Part model, mm, in its own coordinate system. Coordinates: 2 decimals unless noted, no trailing zeros. Order: outer loops, then holes, each group sorted by start corner. A loop starts at its lowest first (then second) coordinate and runs counter-clockwise, first axis right, second up.
1) Cut at C-C (x = -89.5). List the corners of the cut face in (y, z), and give its area (3 significant figures).
2) Wall check: L1, parallel to X at y = 0.4, z = 13.5; L2, parallel to X at y = 2.1, z = -13.5; L3, parallel to X at y = 2.65, z = 7. Give the ranges that are in metal, low to high.
3) Pin check, flat tips, straight feed: pin 1 Ø1.5 at (x, y) = (-113, 2) entering from +Z; pin 2 Ø12 at (x, z) = (-74.5, -11.5) entering from -Y; pin 3 Ø3 at (x, z) = (-105.57, -13.5) entering from +Y; pin 4 Ø1 at (y, z) = (1.5, -20) entering from -X. Stop position of each tip, or through.
4) Cut at A-A (z = -4.5). List the corners of the cut face in (x, y), and give its area (3 significant figures).
5) Cut at B-B (y = 1.8). Give the number of separate pieces and of enclosed holes in the cut face, and give its area (3 significant figures).
```python
from build123d import *

# Parameters (mm, degrees)
EXTRUDE_1_DEPTH              = 3
CUT_EXTRUDE_1_REACH          = 217.134
HOLE_WIZARD_M2_2_D           = 2.4
HOLE_WIZARD_M2_2_CBORE_D     = 4.4
HOLE_WIZARD_M2_2_CBORE_DEPTH = 2
CUT_EXTRUDE_2_REACH          = 217.134
HOLE_WIZARD_M2_3_D           = 2.4
HOLE_WIZARD_M2_3_CBORE_D     = 4.4
HOLE_WIZARD_M2_3_CBORE_DEPTH = 2
MIRROR_7_COPY_1_REACH        = 217.134
MIRROR_7_COPY_2_D            = 2.4
MIRROR_7_COPY_2_CBORE_D      = 4.4
MIRROR_7_COPY_2_CBORE_DEPTH  = 2
CUT_EXTRUDE_3_REACH          = 217.134
SKETCH_18_W                  = 20
SKETCH_18_H                  = 10
HOLE_WIZARD_M2_4_D           = 2.4
HOLE_WIZARD_M2_4_CBORE_D     = 4.4
HOLE_WIZARD_M2_4_CBORE_DEPTH = 2
HOLE_WIZARD_M2_5_D           = 2.4
HOLE_WIZARD_M2_5_CBORE_D     = 4.4
HOLE_WIZARD_M2_5_CBORE_DEPTH = 2
HOLE_WIZARD_M2_6_D           = 2.4
HOLE_WIZARD_M2_6_CBORE_D     = 4.4
HOLE_WIZARD_M2_6_CBORE_DEPTH = 2
SKETCH_24_W                  = 20
SKETCH_24_H                  = 56
CUT_EXTRUDE_4_DEPTH          = 10
HOLE_WIZARD_M2_7_D           = 2.4
HOLE_WIZARD_M2_7_CBORE_D     = 4.4
HOLE_WIZARD_M2_7_CBORE_DEPTH = 2
SKETCH_26_OUTSIDE_W          = 390.69
SKETCH_26_OUTSIDE_H          = 393.83
SKETCH_26_OUTSIDE_W_2        = 151.320508076
SKETCH_26_OUTSIDE_H_2        = 56
CUT_EXTRUDE_6_DEPTH          = 10


with BuildPart() as part:
    # 草图1 → 凸台-拉伸1 (new body)
    with BuildSketch(Plane(origin=(0, 0, 0), x_dir=(1, 0, 0), z_dir=(0, 1, 0))):
        Polygon((-45.715728753, 114), (45.715728753, 114), (84.606601718, 152.890872965), (91.67766953, 152.890872965), (112.890872965, 131.67766953), (112.890872965, 124.606601718), (74, 85.715728753), (74, 30), (91.320508076, 20), (146.320508076, 20), (151.320508076, 15), (151.320508076, -15), (146.320508076, -20), (91.320508076, -20), (74, -30), (74, -85.715728753), (112.890872965, -124.606601718), (112.890872965, -131.67766953), (91.67766953, -152.890872965), (84.606601718, -152.890872965), (45.715728753, -114), (-45.715728753, -114), (-84.606601718, -152.890872965), (-91.67766953, -152.890872965), (-112.890872965, -131.67766953), (-112.890872965, -124.606601718), (-74, -85.715728753), (-74, -30), (-91.320508076, -20), (-146.320508076, -20), (-151.320508076, -15), (-151.320508076, 15), (-146.320508076, 20), (-91.320508076, 20), (-74, 30), (-74, 85.715728753), (-112.890872965, 124.606601718), (-112.890872965, 131.67766953), (-91.67766953, 152.890872965), (-84.606601718, 152.890872965), align=None)
    extrude(amount=EXTRUDE_1_DEPTH)

    # 草图2 → 切除-拉伸1 (cut, up to next)
    with BuildSketch(Plane(origin=(0, 3, 0), x_dir=(1, 0, 0), z_dir=(0, 1, 0)), mode=Mode.PRIVATE) as cut_extrude_1_sk1:
        with BuildLine():
            Line((103.820508076, -10), (103.820508076, 10))
            Line((103.820508076, 10), (129.687258495, 10))
            ThreePointArc((129.687258495, 10), (148.320508076, 0), (129.687258495, -10))
            Line((129.687258495, -10), (103.820508076, -10))
        make_face()
    cut_extrude_1_tool1 = extrude(cut_extrude_1_sk1.sketch, amount=-CUT_EXTRUDE_1_REACH, mode=Mode.PRIVATE) & part.part
    cut_extrude_1 = cut_extrude_1_tool1.solids().sort_by_distance((125.74589, 3, 0))[0]
    add(cut_extrude_1, mode=Mode.SUBTRACT)

    # M2 凹头盖螺钉的柱形沉头孔2 (through all)
    with Locations(Plane(origin=(100.320508076, 3, -8), x_dir=(0, 0, 1), z_dir=(0, 1, 0))):
        with Locations((0, 0), (-5.5, 5.25), (-5.5, 13.25), (-5.5, 21.25), (-5.5, 29.25), (16, 0), (21.5, 5.25), (21.5, 13.25), (21.5, 21.25), (21.5, 29.25)):
            hole_wizard_m2_2 = CounterBoreHole(HOLE_WIZARD_M2_2_D / 2, HOLE_WIZARD_M2_2_CBORE_D / 2, HOLE_WIZARD_M2_2_CBORE_DEPTH)

    # 草图10 → 切除-拉伸2 (cut, up to next)
    with BuildSketch(Plane(origin=(0, 3, 0), x_dir=(1, 0, 0), z_dir=(0, 1, 0)), mode=Mode.PRIVATE) as cut_extrude_2_sk1:
        with BuildLine():
            Line((75.767766953, 101.625631329), (61.625631329, 115.767766953))
            Line((61.625631329, 115.767766953), (79.916185958, 134.058321582))
            ThreePointArc((79.916185958, 134.058321582), (100.162950904, 140.162950904), (94.058321582, 119.916185958))
            Line((94.058321582, 119.916185958), (75.767766953, 101.625631329))
        make_face()
    cut_extrude_2_tool1 = extrude(cut_extrude_2_sk1.sketch, amount=-CUT_EXTRUDE_2_REACH, mode=Mode.PRIVATE) & part.part
    cut_extrude_2 = cut_extrude_2_tool1.solids().sort_by_distance((84.200285, 3, -124.200285))[0]
    add(cut_extrude_2, mode=Mode.SUBTRACT)

    # M2 凹头盖螺钉的柱形沉头孔3 (through all)
    with Locations(Plane(origin=(60.388194462, 3, -119.480077554), x_dir=(0, 0, 1), z_dir=(0, 1, 0))):
        with Locations((0, 0), (-5.65685425, 5.65685425), (-11.313708499, 11.313708499), (-16.970562749, 16.970562749), (7.601397898, 0.176776695), (18.915106397, 11.490485194), (19.091883092, 19.091883092), (13.435028842, 24.748737342), (7.778174593, 30.405591591), (2.121320343, 36.062445841)):
            hole_wizard_m2_3 = CounterBoreHole(HOLE_WIZARD_M2_3_D / 2, HOLE_WIZARD_M2_3_CBORE_D / 2, HOLE_WIZARD_M2_3_CBORE_DEPTH)

    # 镜向5: 切除-拉伸1, M2 凹头盖螺钉的柱形沉头孔2 across plane
    add(cut_extrude_1.mirror(Plane(origin=(0, 0, 0), x_dir=(0, 0, 1), z_dir=(1, 0, 0))), mode=Mode.SUBTRACT)
    add(hole_wizard_m2_2.mirror(Plane(origin=(0, 0, 0), x_dir=(0, 0, 1), z_dir=(1, 0, 0))), mode=Mode.SUBTRACT)

    # 镜向6: 切除-拉伸2, M2 凹头盖螺钉的柱形沉头孔3 across plane
    add(cut_extrude_2.mirror(Plane(origin=(0, 0, 0), x_dir=(0, 0, 1), z_dir=(1, 0, 0))), mode=Mode.SUBTRACT)
    add(hole_wizard_m2_3.mirror(Plane(origin=(0, 0, 0), x_dir=(0, 0, 1), z_dir=(1, 0, 0))), mode=Mode.SUBTRACT)

    # 镜向7: 切除-拉伸2, M2 凹头盖螺钉的柱形沉头孔3 across plane
    add(cut_extrude_2.mirror(Plane.XY), mode=Mode.SUBTRACT)
    add(hole_wizard_m2_3.mirror(Plane.XY), mode=Mode.SUBTRACT)

    # 镜向7 copy 1 sketch → 镜向7 copy 1 (cut, up to next)
    with BuildSketch(Plane(origin=(0, 3, 0), x_dir=(-1, 0, 0), z_dir=(0, 1, 0)), mode=Mode.PRIVATE) as mirror_7_copy_1_sk1:
        with BuildLine():
            Line((75.767766953, 101.625631329), (61.625631329, 115.767766953))
            Line((61.625631329, 115.767766953), (79.916185958, 134.058321582))
            ThreePointArc((79.916185958, 134.058321582), (100.162950904, 140.162950904), (94.058321582, 119.916185958))
            Line((94.058321582, 119.916185958), (75.767766953, 101.625631329))
        make_face()
    mirror_7_copy_1_tool1 = extrude(mirror_7_copy_1_sk1.sketch, amount=-MIRROR_7_COPY_1_REACH, mode=Mode.PRIVATE) & part.part
    add(mirror_7_copy_1_tool1.solids().sort_by_distance((-84.200285, 3, 124.200285))[0], mode=Mode.SUBTRACT)

    # 镜向7 copy 2 (through all)
    with Locations(Plane(origin=(-60.388194462, 3, 119.480077554), x_dir=(0, 0, -1), z_dir=(0, 1, 0))):
        with Locations((0, 0), (-5.65685425, 5.65685425), (-11.313708499, 11.313708499), (-16.970562749, 16.970562749), (7.601397898, 0.176776695), (18.915106397, 11.490485194), (19.091883092, 19.091883092), (13.435028842, 24.748737342), (7.778174593, 30.405591591), (2.121320343, 36.062445841)):
            CounterBoreHole(MIRROR_7_COPY_2_D / 2, MIRROR_7_COPY_2_CBORE_D / 2, MIRROR_7_COPY_2_CBORE_DEPTH)

    # 草图18 → 切除-拉伸3 (cut, up to next)
    with BuildSketch(Plane(origin=(0, 3, 0), x_dir=(1, 0, 0), z_dir=(0, 1, 0)), mode=Mode.PRIVATE) as cut_extrude_3_sk1:
        Polygon((-60, -28), (-15, -28), (-15, -63), (-60, -83), align=None)
    cut_extrude_3_tool1 = extrude(cut_extrude_3_sk1.sketch, amount=-CUT_EXTRUDE_3_REACH, mode=Mode.PRIVATE) & part.part
    # 草图18 → 切除-拉伸3 (cut, up to next)
    with BuildSketch(Plane(origin=(0, 3, 0), x_dir=(1, 0, 0), z_dir=(0, 1, 0)), mode=Mode.PRIVATE) as cut_extrude_3_sk2:
        with Locations((20, -99)):
            Rectangle(SKETCH_18_W, SKETCH_18_H)
    cut_extrude_3_tool2 = extrude(cut_extrude_3_sk2.sketch, amount=-CUT_EXTRUDE_3_REACH, mode=Mode.PRIVATE) & part.part
    # 草图18 → 切除-拉伸3 (cut, up to next)
    with BuildSketch(Plane(origin=(0, 3, 0), x_dir=(1, 0, 0), z_dir=(0, 1, 0)), mode=Mode.PRIVATE) as cut_extrude_3_sk3:
        with Locations((-20, -99)):
            Rectangle(SKETCH_18_W, SKETCH_18_H)
    cut_extrude_3_tool3 = extrude(cut_extrude_3_sk3.sketch, amount=-CUT_EXTRUDE_3_REACH, mode=Mode.PRIVATE) & part.part
    # 草图18 → 切除-拉伸3 (cut, up to next)
    with BuildSketch(Plane(origin=(0, 3, 0), x_dir=(1, 0, 0), z_dir=(0, 1, 0)), mode=Mode.PRIVATE) as cut_extrude_3_sk4:
        Polygon((15, -63), (60, -83), (60, -28), (15, -28), align=None)
    cut_extrude_3_tool4 = extrude(cut_extrude_3_sk4.sketch, amount=-CUT_EXTRUDE_3_REACH, mode=Mode.PRIVATE) & part.part
    # 草图18 → 切除-拉伸3 (cut, up to next)
    with BuildSketch(Plane(origin=(0, 3, 0), x_dir=(1, 0, 0), z_dir=(0, 1, 0)), mode=Mode.PRIVATE) as cut_extrude_3_sk5:
        with Locations((-20, 99)):
            Rectangle(SKETCH_18_W, SKETCH_18_H)
    cut_extrude_3_tool5 = extrude(cut_extrude_3_sk5.sketch, amount=-CUT_EXTRUDE_3_REACH, mode=Mode.PRIVATE) & part.part
    # 草图18 → 切除-拉伸3 (cut, up to next)
    with BuildSketch(Plane(origin=(0, 3, 0), x_dir=(1, 0, 0), z_dir=(0, 1, 0)), mode=Mode.PRIVATE) as cut_extrude_3_sk6:
        with Locations((20, 99)):
            Rectangle(SKETCH_18_W, SKETCH_18_H)
    cut_extrude_3_tool6 = extrude(cut_extrude_3_sk6.sketch, amount=-CUT_EXTRUDE_3_REACH, mode=Mode.PRIVATE) & part.part
    # 草图18 → 切除-拉伸3 (cut, up to next)
    with BuildSketch(Plane(origin=(0, 3, 0), x_dir=(1, 0, 0), z_dir=(0, 1, 0)), mode=Mode.PRIVATE) as cut_extrude_3_sk7:
        Polygon((15, 63), (60, 83), (60, 28), (15, 28), align=None)
    cut_extrude_3_tool7 = extrude(cut_extrude_3_sk7.sketch, amount=-CUT_EXTRUDE_3_REACH, mode=Mode.PRIVATE) & part.part
    # 草图18 → 切除-拉伸3 (cut, up to next)
    with BuildSketch(Plane(origin=(0, 3, 0), x_dir=(1, 0, 0), z_dir=(0, 1, 0)), mode=Mode.PRIVATE) as cut_extrude_3_sk8:
        Polygon((-15, 28), (-15, 63), (-60, 83), (-60, 28), align=None)
    cut_extrude_3_tool8 = extrude(cut_extrude_3_sk8.sketch, amount=-CUT_EXTRUDE_3_REACH, mode=Mode.PRIVATE) & part.part
    add(cut_extrude_3_tool1.solids().sort_by_distance((-39.166667, 3, 50.87037))[0], mode=Mode.SUBTRACT)
    add(cut_extrude_3_tool2.solids().sort_by_distance((20, 3, 99))[0], mode=Mode.SUBTRACT)
    add(cut_extrude_3_tool3.solids().sort_by_distance((-20, 3, 99))[0], mode=Mode.SUBTRACT)
    add(cut_extrude_3_tool4.solids().sort_by_distance((39.166667, 3, 50.87037))[0], mode=Mode.SUBTRACT)
    add(cut_extrude_3_tool5.solids().sort_by_distance((-20, 3, -99))[0], mode=Mode.SUBTRACT)
    add(cut_extrude_3_tool6.solids().sort_by_distance((20, 3, -99))[0], mode=Mode.SUBTRACT)
    add(cut_extrude_3_tool7.solids().sort_by_distance((39.166667, 3, -50.87037))[0], mode=Mode.SUBTRACT)
    add(cut_extrude_3_tool8.solids().sort_by_distance((-39.166667, 3, -50.87037))[0], mode=Mode.SUBTRACT)

    # M2 凹头盖螺钉的柱形沉头孔4 (through all)
    with Locations(Plane(origin=(-20, 3, 109), x_dir=(0, 0, 1), z_dir=(0, 1, 0))):
        with Locations((0, 0), (0, 40), (-218, 0), (-218, 40)):
            CounterBoreHole(HOLE_WIZARD_M2_4_D / 2, HOLE_WIZARD_M2_4_CBORE_D / 2, HOLE_WIZARD_M2_4_CBORE_DEPTH)

    # M2 凹头盖螺钉的柱形沉头孔5 (through all)
    with Locations(Plane(origin=(-69, 3, -40), x_dir=(0, 0, 1), z_dir=(0, 1, 0))):
        with Locations((0, 0), (0, 138)):
            hole_wizard_m2_5 = CounterBoreHole(HOLE_WIZARD_M2_5_D / 2, HOLE_WIZARD_M2_5_CBORE_D / 2, HOLE_WIZARD_M2_5_CBORE_DEPTH)

    # 镜向8: M2 凹头盖螺钉的柱形沉头孔5 across plane
    add(hole_wizard_m2_5.mirror(Plane.XY), mode=Mode.SUBTRACT)

    # M2 凹头盖螺钉的柱形沉头孔6 (through all)
    with Locations(Plane(origin=(-69, 3, 0), x_dir=(0, 0, 1), z_dir=(0, 1, 0))):
        with Locations((0, 0), (0, 138)):
            CounterBoreHole(HOLE_WIZARD_M2_6_D / 2, HOLE_WIZARD_M2_6_CBORE_D / 2, HOLE_WIZARD_M2_6_CBORE_DEPTH)

    # 草图24 → 切除-拉伸4 (cut)
    with BuildSketch(Plane(origin=(0, 3, 0), x_dir=(1, 0, 0), z_dir=(0, 1, 0))):
        Rectangle(SKETCH_24_W, SKETCH_24_H)
    extrude(amount=-CUT_EXTRUDE_4_DEPTH, mode=Mode.SUBTRACT)

    # M2 凹头盖螺钉的柱形沉头孔7 (through all)
    with Locations(Plane(origin=(-20, 3, 0), x_dir=(0, 0, 1), z_dir=(0, 1, 0))):
        with Locations((0, 0), (0, 40)):
            CounterBoreHole(HOLE_WIZARD_M2_7_D / 2, HOLE_WIZARD_M2_7_CBORE_D / 2, HOLE_WIZARD_M2_7_CBORE_DEPTH)

    # 草图26 outside → 切除-拉伸6 (cut)
    with BuildSketch(Plane(origin=(0, 3, 0), x_dir=(1, 0, 0), z_dir=(0, 1, 0))):
        Rectangle(SKETCH_26_OUTSIDE_W, SKETCH_26_OUTSIDE_H)
        with Locations((-75.660254038, 0)):
            Rectangle(SKETCH_26_OUTSIDE_W_2, SKETCH_26_OUTSIDE_H_2, mode=Mode.SUBTRACT)
    extrude(amount=-CUT_EXTRUDE_6_DEPTH, mode=Mode.SUBTRACT)


solid = part.part
```
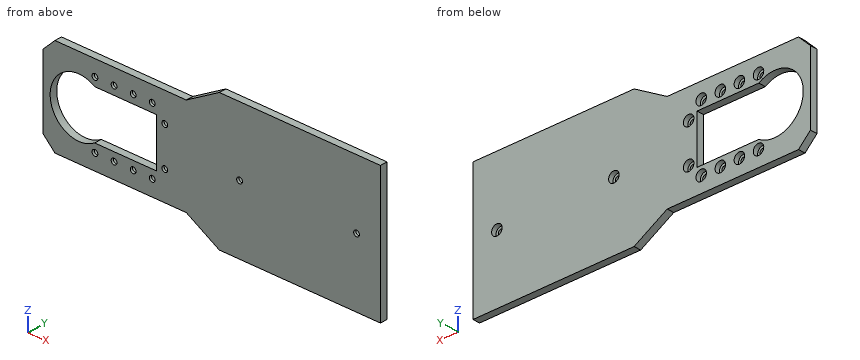
Geometry check:
1. outline: (0, -21.05) - (3, -21.05) - (3, 21.05) - (0, 21.05) - close
1. area: 126 mm2
2. L1: x = -151.32 to -130.77, -128.37 to -122.77, -120.37 to -114.77, -112.37 to -106.77, -104.37 to -10
2. L2: x = -151.32 to -131.77, -127.37 to -123.77, -119.37 to -115.77, -111.37 to -107.77, -103.37 to -10
2. L3: x = -151.32 to -146.07, -103.82 to -102.28, -98.36 to -10
3. pin 1: stops at z = 20
3. pin 2: stops at y = 0
3. pin 3: stops at y = 1
3. pin 4: stops at x = -146.82
4. outline: (-151.32, 0) - (-147.44, 0) - (-147.44, 3) - (-151.32, 3) - close; (-103.82, 0) - (-10, 0) - (-10, 3) - (-103.82, 3) - close
4. area: 293 mm2
5. separate pieces: 1
5. enclosed holes: 13
5. area: 5,740 mm2
